```python
from build123d import *

# Parameters (mm, degrees)
F1_DEPTH = 3
F2_W     = 2
F2_H     = 3
F3_DEPTH = 20
F4_ANGLE = -90


with BuildPart() as f1:
    # F0 (on Top) → F1 (new body)
    with BuildSketch(Plane.XY):
        with BuildLine():
            Line((29.811265, 0), (-28.87221, 0))
            ThreePointArc((-28.87221, 0), (-30.177472, 0.085551), (-31.460401, 0.340742))
            Line((-31.460401, 0.340742), (-49.703157, 5.228874))
            ThreePointArc((-49.703157, 5.228874), (-55.826882, 1.69334), (-52.291348, -4.430385))
            Line((-52.291348, -4.430385), (-33.412757, -9.488888))
            ThreePointArc((-33.412757, -9.488888), (-32.129829, -9.744078), (-30.824567, -9.82963))
            Line((-30.824567, -9.82963), (49.811265, -9.82963))
            Line((49.811265, -9.82963), (49.811265, 25))
            Line((49.811265, 25), (-0.188735, 25))
            ThreePointArc((-0.188735, 25), (-5.188735, 20), (-0.188735, 15))
            Line((-0.188735, 15), (29.811265, 15))
            Line((29.811265, 15), (29.811265, 0))
        make_face()
    extrude(amount=F1_DEPTH)

    # F2 (on face) → F3 (join, through all)
    with BuildSketch(Plane.YZ.offset(49.811265)):
        Polygon((25, -49), (25, 0), (23, 0), (23, -47), (16.384248, -47), (16.384248, -49), align=None)
        with Locations((6.5, -1.5)):
            Rectangle(F2_W, F2_H)
        Polygon((-9.82963, 3), (-6.82963, 3), (-6.82963, 9), (-4.501271, 9), (-4.501271, 12), (-9.82963, 12), align=None)
    extrude(amount=-F3_DEPTH)


with BuildPart() as f1_1:
    # F4: moved
    add(f1.part.rotate(Axis((49.811265, 9.085185, 3), (0, -1, 0)), F4_ANGLE))


solid = f1_1.part
```
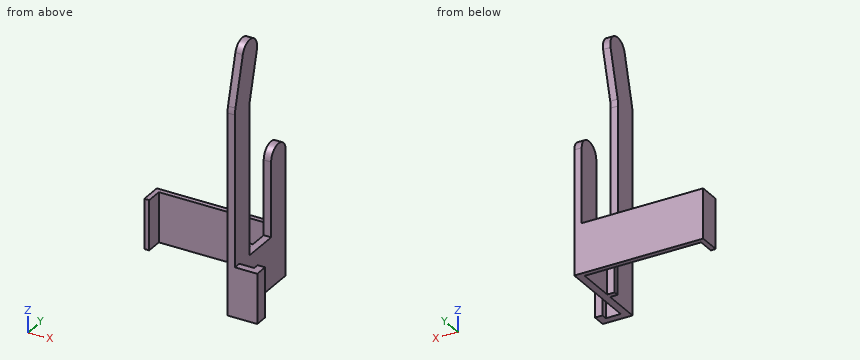
Build history of the part. All positions in model axes, mm. Give positions to 0.01 mm unless a question says otherwise; leave off trailing zeros. Loops run counter-clockwise (first coordinate to the right, second up) from the corner with the lowest first, then second, coordinate; pieces in that order, holes last. Notation, with made-up numbers: (35.5, 66.5) -> (89.5, 66.5) arc R22 ccw to (89.5, 103.5) -> close; hole circle Ø7 at (-29.75, -9.5). An arc over 180 degrees is marked (long way). One line per question, with ' | ' between items. Start each with the question number.
1) Pin check, flat tips, straight feed: pin 1 (3 mm diameter, centred on x = 52, z = 9, fed in from +Y); pin 2 (12 mm diameter, centred on x = 51, z = 44.5, fed in from -Y); pin 3 (6.5 mm diameter, centred on x = 46, y = 7, fed in from +Z); pin 4 (10 mm diameter, centred on y = 5.5, z = 54, fed in from +X). Stop position of each tip, or through.
2) Cut at C-C (x = 30). Give the cut face in (y, z), plus the area to 3 significant figures.
3) Cut at B-B (z = 48). Give the cut face in (x, y).
4) Cut at A-A (y = 20). Give the cut face in (x, z), plus the area to 3 significant figures.
5) Probe L1, parallel to X at y = -1, z = 84; L2, parallel to Y at x = 9, z = 8; L3, parallel to Z at x = 30, y = 23.5. List the from-to ranges inside material, lowest first.
Return value:
1) pin 1: y = -6.83 | pin 2: y = -9.83 | pin 3: z = 107.42 | pin 4: through
2) outline: (23, 3) -> (25, 3) -> (25, 23) -> (23, 23) -> close | area: 40.0 mm^2
3) outline: (46.81, -9.83) -> (49.81, -9.83) -> (49.81, 0) -> (46.81, 0) -> close; (46.81, 15) -> (49.81, 15) -> (49.81, 25) -> (46.81, 25) -> close
4) outline: (-2.19, 3) -> (-0.19, 3) -> (-0.19, 23) -> (-2.19, 23) -> close; (46.81, 3) -> (49.81, 3) -> (49.81, 58) -> (46.81, 58) -> close | area: 205 mm^2
5) L1: 46.81 to 49.81 | L2: 23 to 25 | L3: 3 to 23
